Model file for the job. Use its own axes, mm. Coordinates: 2 decimals unless noted, no trailing zeros. Loops run counter-clockwise (first coordinate to the right, second up) from the corner with the lowest first, then second, coordinate; pieces in that order, holes last.
from build123d import *

# Parameters (mm, degrees)
F0_R     = 10
F1_DEPTH = 20
F3_D     = 15
F3_DEPTH = 10.4935
F3_TIP   = 4.5064546427
F4_R     = 10
F4_R_2   = 8.75
F5_DEPTH = 22
F6_R     = 10
F6_R_2   = 8.64
F7_DEPTH = 18
F8_SIZE  = 0.5


with BuildPart() as f1:
    # F0 (on Front) → F1 (new body, symmetric)
    with BuildSketch(Plane.XZ):
        Circle(F0_R)
    extrude(amount=F1_DEPTH, both=True)

    # F3
    with Locations(Plane.XZ.offset(20)):
        with Locations((0, 0)):
            Hole(F3_D / 2, depth=F3_DEPTH)
            with Locations((0, 0, -(F3_DEPTH + F3_TIP / 2))):  # 118° drill point
                Cone(0, F3_D / 2, F3_TIP, mode=Mode.SUBTRACT)

    # F4 (on face) → F5 (join)
    with BuildSketch(Plane.XZ.offset(20)):
        Circle(F4_R)
        Circle(F4_R_2, mode=Mode.SUBTRACT)
    extrude(amount=F5_DEPTH)

    # F6 (on face) → F7 (join)
    with BuildSketch(Plane.XZ.offset(42)):
        Circle(F6_R)
        Circle(F6_R_2, mode=Mode.SUBTRACT)
    extrude(amount=F7_DEPTH)

    # F8
    f8_edges = [f1.edges().sort_by_distance(p)[0] for p in [
        (-8.64, -60, 0),
        (-10, 20, 0),
    ]]
    chamfer(f8_edges, length=F8_SIZE)


solid = f1.part
Q1. Mould opens along X. For faces 1 (the cylindrical face through (-6.944, -30.846, -5.324)), 2 (the flat face through (9, -60, -3)), 3 (the cylindrical face through (-2.17, -19.69, -9.76)) say: +X half, -X half, draft (parallel to the pull), parting line (faces both ways), or undercut.
Answers:
face 1: undercut
face 2: draft
face 3: parting line
Q2. Slice it at B-B (y = -12). List the corners of the cut face in (x, z), and give its area (3 significant figures).
Answers:
outline: circle Ø20 at (0, 0); hole circle Ø15 at (0, 0)
area: 137 mm2
Q3. Slice it at A-A (y = -34). List the corners of the cut face in (x, z), and give its area (3 significant figures).
Answers:
outline: circle Ø20 at (0, 0); hole circle Ø17.5 at (0, 0)
area: 73.6 mm2
Q4. Drill centre lines: line 1 (Z direction, x = 0, y = -26.75); line 2 (Z direction, x = -0.25, y = -14). Where is each one in solid material? Low to high.
Answers:
line 1: z = -10 to -8.75, 8.75 to 10
line 2: z = -10 to -7.5, 7.5 to 10
Q5. Flat gauge pins, fed straight in: P1, Ø5, axis at x = 3.5, z = 1.5, coming from the -Y side; P2, Ø4, axis at y = -39, z = -2, coming from the +X side; P3, Ø1, axis at x = 7, y = -42, coming from the +Z side; P4, Ø2, axis at y = -33.5, z = 7.5, coming from the +X side. Where does each tip first touch, or does it go through?
Answers:
P1: stops at y = -8.79
P2: stops at x = 10
P3: stops at z = 7.6
P4: stops at x = 7.6
